```python
from build123d import *

# Parameters (mm, degrees)
SKETCH_W        = 20
SKETCH_H        = 20
SKETCH_R        = 1.6
PAD_DEPTH       = 3
PAD001_DEPTH    = 20
SKETCH002_R     = 1.6
POCKET_DEPTH    = 4.561
SKETCH003_W     = 20
SKETCH003_H     = 3
PAD002_DEPTH    = 12.5
SKETCH005_R     = 1.6
POCKET002_DEPTH = 20.001
POCKET003_DEPTH = 20.001
SKETCH006_W     = 20
SKETCH006_H     = 4.5
PAD003_DEPTH    = 3.5
POCKET004_DEPTH = 20.001
SKETCH008_R     = 2.75
POCKET005_DEPTH = 12.501
PAD004_DEPTH    = 20
SKETCH010_R     = 1.6
POCKET006_DEPTH = 17.061
FILLET_R        = 9


with BuildPart() as part:
    # Sketch → Pad (new body)
    with BuildSketch(Plane.XY):
        Rectangle(SKETCH_W, SKETCH_H)
        with Locations((-5.286, 0)):
            Circle(SKETCH_R, mode=Mode.SUBTRACT)
        with Locations((5.286, 0)):
            Circle(SKETCH_R, mode=Mode.SUBTRACT)
    extrude(amount=PAD_DEPTH)

    # Sketch001 (on Face1 of Pad) → Pad001 (join)
    with BuildSketch(Plane(origin=(0, 10, 0), x_dir=(-1, 0, 0), z_dir=(0, 1, 0))):
        Polygon((0, 3), (-4.74, 3), (-2.94, 4.56), (2.94, 4.56), (4.74, 3), align=None)
    extrude(amount=-PAD001_DEPTH)

    # Sketch002 (on Face4 of Pad001) → Pocket (cut, through all)
    with BuildSketch(Plane(origin=(0, 0, 0), x_dir=(1, 0, 0), z_dir=(0, 0, -1))):
        with Locations((-5.286, 0)):
            Circle(SKETCH002_R)
        with Locations((5.286, 0)):
            Circle(SKETCH002_R)
    extrude(amount=-POCKET_DEPTH, mode=Mode.SUBTRACT)

    # Sketch003 (on Face4 of Pocket) → Pad002 (join)
    with BuildSketch(Plane(origin=(0, 0, 0), x_dir=(1, 0, 0), z_dir=(0, 0, -1))):
        with Locations((0, 8.5)):
            Rectangle(SKETCH003_W, SKETCH003_H)
        with Locations((0, -8.5)):
            Rectangle(SKETCH003_W, SKETCH003_H)
    extrude(amount=PAD002_DEPTH)

    # Sketch005 → Pocket002 (cut, through all)
    with BuildSketch(Plane(origin=(0, 10, 0), x_dir=(-1, 0, 0), z_dir=(0, 1, 0))):
        with Locations((0, -8.25)):
            Circle(SKETCH005_R)
    extrude(amount=-POCKET002_DEPTH, mode=Mode.SUBTRACT)

    # Pocket002 Face22 → Pocket003 (cut, through all)
    with BuildSketch(Plane(origin=(0, -10, 3.719063), x_dir=(-1, 0, 0), z_dir=(0, -1, 0))):
        Polygon((-4.74, 0.719063), (-2.94, -0.840937), (2.94, -0.840937), (4.74, 0.719063), (0, 0.719063), align=None)
    extrude(amount=-POCKET003_DEPTH, mode=Mode.SUBTRACT)

    # Sketch006 (on Face11 of Pocket003) → Pad003 (join)
    with BuildSketch(Plane(origin=(0, 0, 0), x_dir=(1, 0, 0), z_dir=(0, 0, -1))):
        with Locations((0, 4.75)):
            Rectangle(SKETCH006_W, SKETCH006_H)
        with Locations((0, -4.75)):
            Rectangle(SKETCH006_W, SKETCH006_H)
    extrude(amount=PAD003_DEPTH)

    # Sketch007 (on Face17 of Pad003) → Pocket004 (cut, through all)
    with BuildSketch(Plane(origin=(-10, 0, 0), x_dir=(0, -1, 0), z_dir=(-1, 0, 0))):
        Polygon((-2.5, 0), (-7, -3.5), (-2.5, -3.5), align=None)
        Polygon((7, -3.5), (2.5, 0), (2.5, -3.5), align=None)
    extrude(amount=-POCKET004_DEPTH, mode=Mode.SUBTRACT)

    # Sketch008 (on Face12 of Pocket004) → Pocket005 (cut, through all)
    with BuildSketch(Plane(origin=(0, 0, 0), x_dir=(1, 0, 0), z_dir=(0, 0, -1))):
        with Locations((-5.286, 0)):
            Circle(SKETCH008_R)
        with Locations((5.286, 0)):
            Circle(SKETCH008_R)
    extrude(amount=POCKET005_DEPTH, mode=Mode.SUBTRACT)

    # Sketch009 (on Face3 of Pocket005) → Pad004 (join)
    with BuildSketch(Plane(origin=(-10, 0, 0), x_dir=(0, -1, 0), z_dir=(-1, 0, 0))):
        Polygon((0, 3), (-4.74, 3), (-2.94, 4.56), (2.94, 4.56), (4.74, 3), align=None)
    extrude(amount=-PAD004_DEPTH)

    # Sketch010 (on Face37 of Pad004) → Pocket006 (cut, through all)
    with BuildSketch(Plane.XY.offset(4.56)):
        with Locations((5.286, 0)):
            Circle(SKETCH010_R)
        with Locations((-5.286, 0)):
            Circle(SKETCH010_R)
    extrude(amount=-POCKET006_DEPTH, mode=Mode.SUBTRACT)

    # Fillet
    fillet_edges = [part.edges().sort_by_distance(p)[0] for p in [
        (-10, -8.5, -12.5),
        (10, 8.5, -12.5),
        (-10, 8.5, -12.5),
        (10, -8.5, -12.5),
    ]]
    fillet(fillet_edges, radius=FILLET_R)


solid = part.part
```
Verification items for the finished model (mm, model axes). A direction names the side the tool comes from. Round coordinates to 2 decimals unless told otherwise and drop trailing zeros. Write each loop counter-clockwise with the first axis right and the second up, starting at its lowest first coordinate (ties: lowest second). Pieces come first, ordered by that corner, then holes.
1. Access from +Z, -Z, +X, -X, +Y, -Y to the whole of each face (thin tool, end or side, straight path). Record for faces 5 (the cylindrical face through (-7.294, 8.479, -9.934)), 6 (the flat face through (0, -7, -6)).
2. Section check D-D on z = -9.5. Enter the section's corners in (x, y), plus the area to 3 significant figures.
3. Section check C-C on z = 0.5. Enter the section's corners in (x, y), plus the area to 3 significant figures.
4. Scan lines: L1, parallel to Y at x = -3.5, z = -4; L2, parallel to Z at x = 0, y = 8.6; L3, parallel to Z at x = 2.75, y = -2. Record each from-to range of solid material in increasing order.
5. Section check A-A on x = 0. Enter the section's corners in (y, z).
6. Draft check along X on faces 1 (the flat face through (-10, 0, 1)), 2 (the cylindrical face through (-6.884, 0.07, 2.248)), 3 (the cylindrical face through (0.35, -8.48, -9.81)), 4 (the flat face through (-0.14, -4.781, -1.774)). Enter one of: +X half, -X half, draft (parallel to the pull), parting line (faces both ways), or undercut.
7. Section check B-B on y = 0. Enter the section's corners in (x, z), plus the area to 3 significant figures.
8. Gauge pin test, flat ends, axial feed: P1, Ø6, axis at x = 3.5, y = -6.5, coming from the +Z side; P2, Ø2, axis at x = 6.5, y = 3, coming from the +Z side; P3, Ø6, axis at x = 3, y = 0, coming from the -Z side; P4, Ø2, axis at x = -3, y = 6.5, coming from the -Z side. Record the tip position at first contact, or that the pin passes through.
Answer:
1. face 5: -Z, -X, +Y, -Y
1. face 6: -Z, +X, -X
2. outline: (-7.71, -10) - (-1, -10) - (-1, -7) - (-7.71, -7) - close; (-7.71, 7) - (-1, 7) - (-1, 10) - (-7.71, 10) - close; (1, -10) - (7.71, -10) - (7.71, -7) - (1, -7) - close; (1, 7) - (7.71, 7) - (7.71, 10) - (1, 10) - close
2. area: 80.5 mm2
3. outline: (-10, -10) - (10, -10) - (10, 10) - (-10, 10) - close; hole circle Ø3.2 at (-5.29, 0); hole circle Ø3.2 at (5.29, 0)
3. area: 384 mm2
4. L1: y = -10 to -7, 7 to 10
4. L2: z = -12.5 to -9.85, -6.65 to 3
4. L3: z = 0 to 4.56
5. outline: (-10, -12.5) - (-7, -12.5) - (-7, -9.85) - (-10, -9.85) - close; (-10, -6.65) - (-7, -6.65) - (-7, -3.5) - (-2.5, 0) - (2.5, 0) - (7, -3.5) - (7, -6.65) - (10, -6.65) - (10, 3) - (4.74, 3) - (2.94, 4.56) - (-2.94, 4.56) - (-4.74, 3) - (-10, 3) - close; (7, -12.5) - (10, -12.5) - (10, -9.85) - (7, -9.85) - close
6. face 1: -X half
6. face 2: undercut
6. face 3: undercut
6. face 4: draft
7. outline: (-10, 0) - (-6.89, 0) - (-6.89, 4.56) - (-10, 4.56) - close; (-3.69, 0) - (3.69, 0) - (3.69, 4.56) - (-3.69, 4.56) - close; (6.89, 0) - (10, 0) - (10, 4.56) - (6.89, 4.56) - close
7. area: 62.0 mm2
8. P1: stops at z = 4.07
8. P2: stops at z = 4.56
8. P3: stops at z = -0.39
8. P4: stops at z = -12.43
